Geometry: final body of the model. Coordinates: model frame, mm. A direction names the side the tool comes from. Round coordinates to 2 decimals unless told otherwise and drop trailing zeros. Loops run counter-clockwise (first coordinate to the right, second up) from the corner with the lowest first, then second, coordinate; pieces in that order, holes last. Notation, with made-up numbers: M 5.25,67 L 47.25,67 A16 ccw 47.25,82 Z; hole C -4.75,60 d10. An arc over 180 degrees is marked long. Answer as a JSON object with one key per item and string values.
```python
from build123d import *

# Parameters (mm, degrees)
ESBO_O1_W                        = 45
ESBO_O1_H                        = 45
RESSALTO_EXTRUS_O1_DEPTH         = 20
ESBO_O2_W                        = 25
ESBO_O2_H                        = 25
CORTE_EXTRUS_O1_DEPTH            = 70.705238631
ESBO_O3_W                        = 20
ESBO_O3_H                        = 20
RESSALTO_EXTRUS_O2_DEPTH         = 25
FURO_DE_DI_METRO_6_2_6_2_1_D     = 6.2
FURO_DE_DI_METRO_6_2_6_2_1_DEPTH = 35
FURO_DE_DI_METRO_6_2_6_2_2_D     = 6.2
FURO_DE_DI_METRO_6_2_6_2_2_DEPTH = 35
FURO_DE_DI_METRO_6_2_6_2_3_D     = 6.2
FURO_DE_DI_METRO_6_2_6_2_3_DEPTH = 35
FILETE2_R                        = 8
CHANFRO1_SIZE                    = 25
CHANFRO2_SIZE                    = 25
RESSALTO_EXTRUS_O3_DEPTH         = 20
ESBO_O12_R                       = 3
CORTE_EXTRUS_O2_DEPTH            = 71.906960985
CORTE_EXTRUS_O5_DEPTH            = 3
CORTE_EXTRUS_O5_DEPTH_BACK       = 3
ESBO_O18_R                       = 3.5
CORTE_EXTRUS_O6_DEPTH            = 69.698424668


# Some blends are built 0.0001 mm under size
with BuildPart() as part:
    # Esboço1 → Ressalto-extrusão1 (new body)
    with BuildSketch(Plane.XY.offset(20)):
        with Locations((-12.862035225, 34.142270059)):
            Rectangle(ESBO_O1_W, ESBO_O1_H)
    extrude(amount=-RESSALTO_EXTRUS_O1_DEPTH)

    # Esboço2 → Corte-extrusão1 (cut, through all)
    with BuildSketch(Plane(origin=(0, 0, 0), x_dir=(-1, 0, 0), z_dir=(0, 0, -1))):
        with Locations((2.862035225, 44.142270059)):
            Rectangle(ESBO_O2_W, ESBO_O2_H)
    extrude(amount=-CORTE_EXTRUS_O1_DEPTH, mode=Mode.SUBTRACT)

    # Esboço3 → Ressalto-extrusão2 (add)
    with BuildSketch(Plane.XY.offset(20)):
        with Locations((-25.362035225, 21.642270059)):
            Rectangle(ESBO_O3_W, ESBO_O3_H)
    extrude(amount=RESSALTO_EXTRUS_O2_DEPTH)

    # Furo de diâmetro Ø6.2 (6.2)1
    with Locations(Plane(origin=(9.637964775, 0, 0), x_dir=(0, 0, -1), z_dir=(1, 0, 0))):
        with Locations((-10, 21.642270059)):
            Hole(FURO_DE_DI_METRO_6_2_6_2_1_D / 2, depth=FURO_DE_DI_METRO_6_2_6_2_1_DEPTH)

    # Furo de diâmetro Ø6.2 (6.2)2
    with Locations(Plane(origin=(0, 56.642270059, 0), x_dir=(1, 0, 0), z_dir=(0, 1, 0))):
        with Locations((-25.362035225, -10)):
            Hole(FURO_DE_DI_METRO_6_2_6_2_2_D / 2, depth=FURO_DE_DI_METRO_6_2_6_2_2_DEPTH)

    # Furo de diâmetro Ø6.2 (6.2)3
    with Locations(Plane.XY.offset(45)):
        with Locations((-25.362035225, 21.642270059)):
            Hole(FURO_DE_DI_METRO_6_2_6_2_3_D / 2, depth=FURO_DE_DI_METRO_6_2_6_2_3_DEPTH)

    # Filete2
    filete2_edges = [part.edges().sort_by_distance(p)[0] for p in [
        (-35.362035225, 34.142270059, 0),
        (-12.862035225, 11.642270059, 0),
        (-35.362035225, 11.642270059, 22.5),
    ]]
    fillet(filete2_edges, radius=FILETE2_R)

    # Chanfro1
    # the kernel refuses this chamfer: 25 mm, written as the material it adds along each edge
    with BuildSketch(Plane(origin=(-35.362035225, 31.642270059, 20), x_dir=(0, -0.027495876610586317, 0.9996219169112966), z_dir=(1, 0, 0))) as chanfro1_piece_1_section:
        Polygon((CHANFRO1_SIZE * 0.999621916911, -CHANFRO1_SIZE * 0.0274958766106), (-CHANFRO1_SIZE * 0.0274958766106, -CHANFRO1_SIZE * 0.999621916911), (0, 0), align=None)
    chanfro1_piece_1 = extrude(amount=20, mode=Mode.PRIVATE)
    chanfro1_piece_1 = split(chanfro1_piece_1, bisect_by=Plane(origin=(-25.362035225, 39.873368248, 45), z_dir=(0, 0, -1)), keep=Keep.TOP, mode=Mode.PRIVATE)
    chanfro1_piece_1 = split(chanfro1_piece_1, bisect_by=Plane(origin=(-25.362035225, 56.642270059, 28.231098189), z_dir=(0, -1, 0)), keep=Keep.TOP, mode=Mode.PRIVATE)
    add(chanfro1_piece_1)

    # Chanfro2
    chanfro2_edges = [part.edges().sort_by_distance(p)[0] for p in [
        (-15.362035225, 31.642270059, 10),
    ]]
    chamfer(chanfro2_edges, length=CHANFRO2_SIZE - 0.0001)  # a hair under: the kernel refuses the full size

    # Esboço10 → Ressalto-extrusão3 (add)
    with BuildSketch(Plane.XZ.offset(-11.642270059)):
        Polygon((-15.362035225, 45), (9.637964775, 20), (-15.362035225, 20), align=None)
    extrude(amount=-RESSALTO_EXTRUS_O3_DEPTH)

    # Esboço12 → Corte-extrusão2 (cut, through all)
    with BuildSketch(Plane(origin=(20.426744945, 20.426744945, 20.426744945), x_dir=(-0.8164965809277259, 0.408248290463863, 0.4082482904638632), z_dir=(-0.577350269189626, -0.5773502691896256, -0.5773502691896258))):
        with Locations(Location((33.625917704, 8.232328107, 0), (0, 0, 120.000005232))):
            Circle(ESBO_O12_R)
    extrude(amount=CORTE_EXTRUS_O2_DEPTH, mode=Mode.SUBTRACT)

    # Esboço16 → Corte-extrusão5 (cut, two sides: drawn at the far end of the back side and taken through both)
    with BuildSketch(Plane(origin=(0, 21.642270059, 0), x_dir=(-1, 0, 0), z_dir=(0, -1, 0)).offset(-CORTE_EXTRUS_O5_DEPTH_BACK)):
        Polygon((10.362035225, -40), (17.262035225, -33.1), (17.262035225, -18.1), (-4.637964775, -18.1), (-4.637964775, -25), align=None)
    extrude(amount=CORTE_EXTRUS_O5_DEPTH + CORTE_EXTRUS_O5_DEPTH_BACK, mode=Mode.SUBTRACT)

    # Esboço18 → Corte-extrusão6 (cut, through all)
    with BuildSketch(Plane(origin=(0, 18.642270059, 0), x_dir=(1, 0, 0), z_dir=(0, 1, 0))):
        with Locations(Location((-8.762035225, -25, 0), (0, 0, 270))):
            Circle(ESBO_O18_R)
    extrude(amount=-CORTE_EXTRUS_O6_DEPTH, mode=Mode.SUBTRACT)


solid = part.part
```
1) First-contact query: pin 1 (3.5 mm diameter, centred on y = 21.64, z = 10, fed in from +X); pin 2 (8 mm diameter, centred on x = -11, z = 32, fed in from +Y); pin 3 (4 mm diameter, centred on x = -15, y = 48, fed in from +Z). Flat tips, straight axial feed; report the tip coordinate or a pass-through.
Geometry results:
{"pin 1": "x = -28.2", "pin 2": "y = 31.64", "pin 3": "z = 30.61"}
2) Pull-direction query (Y, two-part tool) for faces 1 (the face through (-8.6, 14.05, 2.28)), 2 (the face through (-28, 56.642, 12)), 3 (the face through (-17.262, 22, 26)); classes: +Y half, -Y half, draft (parallel to the pull), parting line (faces both ways), or undercut.
Geometry results:
{"face 1": "-Y half", "face 2": "+Y half", "face 3": "undercut"}
3) Cut plane B-B on x = -3.5. Return the cut outline in (y, z), and give its area (3 significant figures).
Geometry results:
{"outline": "M 11.64,8 A8 ccw 19.64,0 L 44.78,0 L 44.78,20 L 31.64,20 L 31.64,33.14 L 24.64,33.14 L 24.64,18.1 L 18.64,18.1 L 18.64,33.14 L 11.64,33.14 Z; hole C 21.64,10 d6.2", "area": "791 mm2"}
4) Cut plane A-A on y = 41. Return the cut outline in (x, z).
Geometry results:
{"outline": "M -35.36,8 A8 ccw -27.36,0 L 0.28,0 L 0.28,20 L -15.36,20 L -15.36,35.64 L -35.36,35.64 Z; hole C -25.36,10 d6.2"}
5) Line query: probe 1 along X at (y, z) = (21.5, 19.5); probe 2 along Y at (x, z) = (-3, 31); probe 3 along Z at (x, y) = (-6, 44). Output: solid intervals per line, ascending.
Geometry results:
{"probe 1": "-35.36 to -28.46, -22.27 to -17.26, 4.64 to 9.64", "probe 2": "11.64 to 18.64, 24.64 to 31.64", "probe 3": "0 to 20"}
6) Set-up query: faces 4 (the face through (-15.362, 40, 29)), 5 (the face through (-28.226, 20.455, 27.58)), 6 (the face through (-27.029, 39.222, 7.386)), 7 (the face through (-6, 22, 18.1)). Return all of +Z, -Z, +X, -X, +Y, -Y with unobstructed straight access to the full face (end or side cutting, diameter ignored); none if empty.
Geometry results:
{"face 4": "+Z, +X, +Y", "face 5": "+Z", "face 6": "+Y", "face 7": "none"}
7) Cut plane C-C on z = 42. Return the cut outline in (x, y).
Geometry results:
{"outline": "M -35.36,19.64 A8 ccw -27.36,11.64 L -12.36,11.64 L -12.36,31.64 L -15.36,31.64 L -15.36,34.64 L -35.36,34.64 Z; hole C -25.36,21.64 d6.2"}
